Autodesk Inventor part; units mm, degrees
ref_plane "YZ Plane" through (0, 0, 0) normal (1, 0, 0) x (0, 1, 0)
ref_plane "XZ Plane" through (0, 0, 0) normal (0, 1, 0) x (-1, 0, 0)
ref_plane "XY Plane" through (0, 0, 0) normal (0, 0, 1) x (1, 0, 0)
sketch "Sketch1" plane through (0, 0, 0) normal (0, 1, 0) x (-1, 0, 0)
  line L0 (0, 0) -> (0, -2.8284)
  line L1 (0, -2.8284) -> (29, 26.1716)
  line L2 (29, 26.1716) -> (29, 29)
  line L3 (29, 29) -> (0, 0)
  line L4 (29, 26.1716) -> (40, 37.1716)
  line L5 (40, 37.1716) -> (40, 40)
  line L6 (40, 40) -> (29, 29)
  dimension "d2" = 29
  dimension "d3" = 45
  dimension "d6" = 2
  dimension "d23" = 11
  dimension "d24" = 45
  dimension "d25" = 45
extrude "Extrusion1" add sketch "Sketch1" along normal mid plane 100 contours L3 L2 L1 L0
sketch "Sketch2" plane through (0, 0, 0) normal (0, 0, 1) x (1, 0, 0)
  line L0 (-17, 36) -> (-6, 36)
  line L1 (-6, 36) -> (-6, 19)
  line L2 (-6, 19) -> (-17, 19)
  line L3 (-17, 19) -> (-17, 36)
  line L4 (0, 50) -> (-29, 50)
  line L5 (0, -50) -> (0, 50)
  point P0 (0, 0)
  dimension "d7" = 14
  dimension "d8" = 17
  dimension "d9" = 11
  dimension "d11" = 6
extrude "Extrusion2" cut sketch "Sketch2" along normal up to next
mirror "Mirror1" about plane through (0, 0, 0) normal (0, 1, 0) of "Extrusion2"
sketch "Sketch3" plane through (0, -50, 0) normal (0.7071, 0, 0.7071) x (0.7071, 0, -0.7071)
  circle A0 centre (-30.5122, 5) radius 1.25
  circle A1 centre (-15.5122, 5) radius 1.25
  line L0 (-39.0122, 0) -> (-39.0122, 100)
  line L1 (-41.0122, 0) -> (-41.0122, 100)
  line L2 (0, 0) -> (-41.0122, 0)
  point P0 (0, 50)
  dimension "d15" = 5
  dimension "d16" = 2.5
  dimension "d17" = 15
  dimension "d18" = 2.5
  dimension "d19" = 5
  dimension "d20" = 10.5
extrude "Extrusion3" cut sketch "Sketch3" against normal up to next
mirror "Mirror2" about plane through (0, 0, 0) normal (0, 1, 0) of "Extrusion3"
extrude "Extrusion4" add sketch "Sketch1" along normal mid plane 100 contours L6 L5 L4 L2
properties part number "Front_Dluzszy_3"
The model under review builds one solid part; all positions refer to its coordinate system, in mm. A direction names the side the tool comes from. Give positions to 0.01 mm unless a question says otherwise; leave off trailing zeros. Write each loop counter-clockwise with the first axis right and the second up, starting at its lowest first coordinate (ties: lowest second). Pieces come first, ordered by that corner, then holes.
(1) Consider section C-C, the plane y = -41. Give the boundary of the cut face in (x, z).
(2) For P1, Ø1.5, axis at y = -0.5, z = 14.5, coming from the +X side; P2, Ø2.5, axis at y = 27, z = 15.5, coming from the +X side; P3, Ø2.5, axis at y = -23.5, z = 5, coming from the -X side; P4, Ø2, axis at y = -27.5, z = 8.5, coming from the +X side, all flat-tipped, find the tip position at first contact; note any pin that passes through.
(3) Tool access review of faces 5 (the flat face through (-6, -27, 5)), 6 (the flat face through (-40, -1, 39)), 7 (the flat face through (-17, 27, 16)): name each direction out of +Z, -Z, +X, -X, +Y, -Y from which nothing blocks a thin tool from reaching the whole face with its end or side.
(4) Consider section B-B, the plane y = 22. Give the boundary of the cut face in (x, z).
(5) Consider section A-A, the plane x = -7.5. Give the boundary of the cut face in (y, z), and give its area (3 significant figures).
(6) The part is to be moulded in two halves that separate along Z. For faces 1 (the flat face through (-20, -1, 20)), 2 (the flat face through (-19.72, -0.7, 16.89)), 3 (the cylindrical face through (-11.78, 46.24, 10.39)), 4 (the flat face through (-17, -28, 16)), say which applies: released by +Z, released by -Z, zero draft, split by the parting line, or undercut.
(7) To check wall thickness, follow L1, parallel to Y at x = -10, z = 9.5; L2, parallel to X at y = -32, z = 19; L3, parallel to X at y = -43, z = 2. State the ranges of each line that lie inside material, in increasing order.
(8) Consider section D-D, the plane z = 1. Give the boundary of the cut face in (x, y), and give its area (3 significant figures).
Returned:
1. outline: (-40, 37.17) - (0, -2.83) - (0, 0) - (-40, 40) - close
2. P1: stops at x = -13.75
2. P2: stops at x = -17
2. P3: stops at x = -6
2. P4: passes through
3. face 5: +Z, -Z, -X
3. face 6: +Z, -Z, -X, +Y, -Y
3. face 7: +Z, -Z, +X
4. outline: (-40, 37.17) - (-17, 14.17) - (-17, 17) - (-40, 40) - close; (-6, 3.17) - (0, -2.83) - (0, 0) - (-6, 6) - close
5. outline: (-50, 4.67) - (-36, 4.67) - (-36, 7.5) - (-50, 7.5) - close; (-19, 4.67) - (19, 4.67) - (19, 7.5) - (-19, 7.5) - close; (36, 4.67) - (50, 4.67) - (50, 7.5) - (36, 7.5) - close
5. area: 187 mm2
6. face 1: released by +Z
6. face 2: released by -Z
6. face 3: undercut
6. face 4: zero draft
7. L1: y = -50 to -36, -19 to 19, 36 to 50
7. L2: x = -21.83 to -19
7. L3: x = -4.83 to -2
8. outline: (-3.83, -50) - (-1, -50) - (-1, 50) - (-3.83, 50) - close
8. area: 283 mm2
